Check sheet for the modelled part. Datum: model origin and axes. Units: mm. A direction names the side the tool comes from. Give positions to 0.01 mm unless a question says otherwise; leave off trailing zeros. Order: outer loops, then holes, each group sorted by start corner. A loop starts at its lowest first (then second) coordinate and runs counter-clockwise, first axis right, second up.
from build123d import *

# Parameters (mm, degrees)
SKETCH1_W           = 16.5
SKETCH1_H           = 18
BOSS_EXTRUDE1_DEPTH = 1.75
SKETCH3_W           = 16.5
SKETCH3_H           = 2.5
BOSS_EXTRUDE2_DEPTH = 6.5
SKETCH2_W           = 4
SKETCH2_H           = 4
BOSS_EXTRUDE3_DEPTH = 2


with BuildPart() as part:
    # Sketch1 → Boss-Extrude1 (new body)
    with BuildSketch(Plane(origin=(0, 0, 0), x_dir=(1, 0, 0), z_dir=(0, 1, 0))):
        Rectangle(SKETCH1_W, SKETCH1_H)
    extrude(amount=BOSS_EXTRUDE1_DEPTH)

    # Sketch3 → Boss-Extrude2 (add)
    with BuildSketch(Plane(origin=(0, 1.75, 0), x_dir=(1, 0, 0), z_dir=(0, 1, 0))):
        with Locations((0, -7.75)):
            Rectangle(SKETCH3_W, SKETCH3_H)
    extrude(amount=BOSS_EXTRUDE2_DEPTH)

    # Sketch2 → Boss-Extrude3 (add)
    with BuildSketch(Plane(origin=(0, 0, 0), x_dir=(1, 0, 0), z_dir=(0, 1, 0))):
        with Locations((0, -1)):
            Rectangle(SKETCH2_W, SKETCH2_H)
    extrude(amount=-BOSS_EXTRUDE3_DEPTH)


solid = part.part
1) Section check C-C, the plane y = 2.5. Record the cut outline in (x, z).
Recorded:
outline: (-8.25, 6.5) - (8.25, 6.5) - (8.25, 9) - (-8.25, 9) - close
2) Depth check by flat-ended pin: pin 1 Ø2 at (x, y) = (0, -1.5) entering from +Z; pin 2 Ø2 at (x, y) = (2.5, 4.5) entering from -Z; pin 3 Ø1 at (x, z) = (-3.5, 5.5) entering from -Y. Enter the tip coordinate at first touch or a pass-through.
Recorded:
pin 1: stops at z = 3
pin 2: stops at z = 6.5
pin 3: stops at y = 0
3) Material ranges on L1, parallel to Z at x = 1, y = 8; L2, parallel to Y at x = 7.5, z = 5; L3, parallel to Y at x = 4.5, z = 7.5, recorded low to high.
Recorded:
L1: z = 6.5 to 9
L2: y = 0 to 1.75
L3: y = 0 to 8.25
4) Set-up check for faces 1 (the face through (-2, -1, 1)), 2 (the face through (0, -1, -1)), 3 (the face through (2, -1, 1)), 4 (the face through (0, -1, 3)), 5 (the face through (0, 5, 6.5)): record each of +Z, -Z, +X, -X, +Y, -Y from which the full face is reachable in a straight line by a thin tool's end or side.
Recorded:
face 1: +Z, -Z, -X, -Y
face 2: -Z, +X, -X, -Y
face 3: +Z, -Z, +X, -Y
face 4: +Z, +X, -X, -Y
face 5: -Z, +X, -X, +Y
5) Section check D-D, the plane x = -6. Record the cut outline in (y, z), then the cut area to 4 significant figures.
Recorded:
outline: (0, -9) - (1.75, -9) - (1.75, 6.5) - (8.25, 6.5) - (8.25, 9) - (0, 9) - close
area: 47.75 mm2
6) Section check A-A, the plane z = -0.25. Record the cut outline in (x, y).
Recorded:
outline: (-8.25, 0) - (-2, 0) - (-2, -2) - (2, -2) - (2, 0) - (8.25, 0) - (8.25, 1.75) - (-8.25, 1.75) - close
7) Section check B-B, the plane x = 1. Record the cut outline in (y, z).
Recorded:
outline: (-2, -1) - (0, -1) - (0, -9) - (1.75, -9) - (1.75, 6.5) - (8.25, 6.5) - (8.25, 9) - (0, 9) - (0, 3) - (-2, 3) - close
